from build123d import *

# Parameters (mm, degrees)
FILLET1_R = 1
SKETCH3_W = 1.25
SKETCH3_H = 8.5


with BuildPart() as part:
    # Sketch1 → Revolve1 (revolve)
    with BuildSketch(Plane.XY):
        Polygon((-8.5, -51.915), (-8.5, -7.915), (-9.5, -7.915), (-9.5, -6.5), (-8.5, -6.5), (-8.5, 0), (-10, 0), (-10, 1.5), (-8.5, 1.5), (-8.5, 13.5), (-10, 13.5), (-10, 15), (0, 15), (0, -37.915), (-4, -37.915), (-4, -51.915), align=None)
    revolve(axis=Axis((0, 15, 0), (0, -1, 0)))

    # Fillet1
    fillet1_edges = [part.edges().sort_by_distance(p)[0] for p in [
        (8.5, -51.915, 0),
        (4, -51.915, 0),
    ]]
    fillet(fillet1_edges, radius=FILLET1_R)

    # Sketch3 → M3x0.5 Tapped Hole1 (revolve, cut)
    with BuildSketch(Plane(origin=(0, -43.915, 0), x_dir=(0, 1, 0), z_dir=(1, 0, 0))):
        with Locations((0.625, 4.25)):
            Rectangle(SKETCH3_W, SKETCH3_H)
    revolve(axis=Axis((0, -43.915, -6.35), (0, 0, 1)), mode=Mode.SUBTRACT)


solid = part.part
Verification items for the finished model (mm, model axes). A direction names the side the tool comes from. Round coordinates to 2 decimals unless told otherwise and drop trailing zeros. Loops run counter-clockwise (first coordinate to the right, second up) from the corner with the lowest first, then second, coordinate; pieces in that order, holes last. Notation, with made-up numbers: (40, 4.5) - (74, 4.5) arc R8 ccw to (74, 17.5) - close; hole circle Ø6 at (21.25, 51). An arc over 180 degrees is marked (long way). Write item = value, one per line.
Q1. Tool access check on faces 4 (the cylindrical face through (-4.38, -7.2, 8.43)), 5 (the cylindrical face through (-0.375, -42.723, 6.183)), 6 (the cylindrical face through (-4.57, -3.204, -7.167)), 7 (the cylindrical face through (2.17, 0.76, 9.76)). Record the directions out of +Z, -Z, +X, -X, +Y, -Y that give a thin tool (end or side, any length) a straight path to the whole face; none if there is none.
Here are the results:
face_4 = -Y
face_5 = +Z
face_6 = none
face_7 = +Y, -Y
Q2. Depth check by flat-ended pin: pin 1 (2.5 mm diameter, centred on x = 1, z = 1, fed in from -Y) (3 decimals); pin 2 (6 mm diameter, centred on x = -7.5, y = -42, fed in from +Z); pin 3 (6 mm diameter, centred on y = 3.5, z = -3.5, fed in from +X). Enter the tip coordinate at first touch or a pass-through.
Here are the results:
pin_1 = -37.915
pin_2 = 7.21
pin_3 = 9.92
Q3. Material ranges on L1, parallel to Y at x = 8.5, z = -3.25 (3 decimals); L2, parallel to Y at x = -7.25, z = 6.75; L3, parallel to Y at x = 0, z = 6.4 (3 decimals), recorded low to high.
Here are the results:
L1 = -7.915 to -6.5, 0 to 1.5, 13.5 to 15
L2 = 0 to 1.5, 13.5 to 15
L3 = -51.915 to -45.165, -42.665 to 15
Q4. Mould release check, pull along Y, two halves, no side actions. Record for faces 1 (the cylindrical face through (2.17, 14.26, 9.76)), 2 (the flat face through (0, -37.915, 0)), 3 (the flat face through (-4.5, 13.5, 7.4)): +Y half, -Y half, draft (parallel to the pull), parting line (faces both ways), or undercut.
Here are the results:
face_1 = draft
face_2 = -Y half
face_3 = undercut
Q5. Sectioned sample at B-B on y = -48. Record the boundary of the cut face in (x, z), plus the area to 3 significant figures.
Here are the results:
outline = circle Ø17 at (0, 0); hole circle Ø8 at (0, 0)
area = 177 mm^2
Q6. Sectioned sample at C-C on y = -34.5. Record the boundary of the cut face in (x, z), plus the area to 3 significant figures.
Here are the results:
outline = circle Ø17 at (0, 0)
area = 227 mm^2
